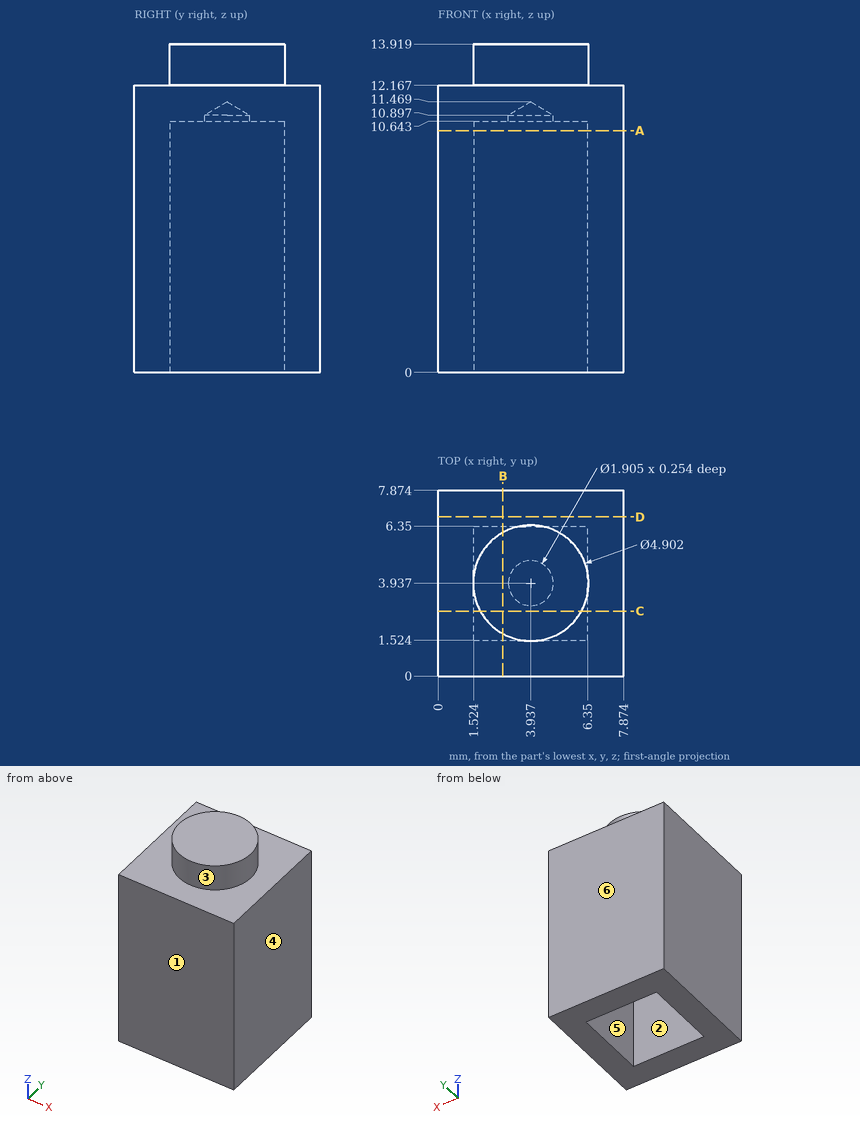
Geometry check sheet. Reference: drawing and pictorial views, mm from the part's lowest x, y, z. A direction names the side the tool comes from. Round coordinates to 2 decimals unless told otherwise and drop trailing zeros. Loops run counter-clockwise (first coordinate to the right, second up) from the corner with the lowest first, then second, coordinate; pieces in that order, holes last. Notation, with made-up numbers: (57.25, 25.5) - (84.25, 25.5) arc R26 ccw to (84.25, 46.5) - close; hole circle Ø1 at (25, 60). An arc over 180 degrees is marked (long way). Write item = value, one per line. Start each with the question number.
Q1. Thickness scan on L1, parallel to X at y = 6, z = 6; L2, parallel to Z at x = 4.5, y = 2. Record the ranges inside material, lowest first.
Q2. Release check for a two-part mould opening along Y. For the marked faces 4, 5 and 6 record: pulls with the +Y half, pulls with the -Y half, needs draft (parallel to the pull), parting line crosses it, or undercut.
Q3. Section check B-B (x = 2.75). Record the boundary of the cut face in (y, z).
Q4. Section check A-A (z = 10.25). Record the boundary of the cut face in (x, y).
Q5. Section check D-D (y = 6.75). Record the boundary of the cut face in (x, z), plus the area to 3 significant figures.
Q6. Access from +Z, -Z, +X, -X, +Y, -Y to the whole of each face (thin tool, end or side, straight path). Record for the marked faces 1, 2 and 3.
Q7. Depth check by flat-ended pin: P1, Ø2.5, axis at x = 3.937, y = 3.937, coming from the -Z side. Enter the tip coordinate at first touch or a pass-through.
Derived:
q1.L1 = 0 to 1.52, 6.35 to 7.87
q1.L2 = 10.64 to 13.92
q2.face_4 = needs draft
q2.face_5 = undercut
q2.face_6 = pulls with the +Y half
q3.outline = (0, 0) - (1.52, 0) - (1.52, 10.64) - (6.35, 10.64) - (6.35, 0) - (7.87, 0) - (7.87, 12.17) - (6.08, 12.17) - (6.08, 13.92) - (1.79, 13.92) - (1.79, 12.17) - (0, 12.17) - close
q4.outline = (0, 0) - (7.87, 0) - (7.87, 7.87) - (0, 7.87) - close; hole (1.52, 1.52) - (6.35, 1.52) - (6.35, 6.35) - (1.52, 6.35) - close
q5.outline = (0, 0) - (7.87, 0) - (7.87, 12.17) - (0, 12.17) - close
q5.area = 95.8 mm^2
q6.face_1 = +Z, -Z, +X, -X, -Y
q6.face_2 = -Z
q6.face_3 = +Z
q7.P1 = 10.64
